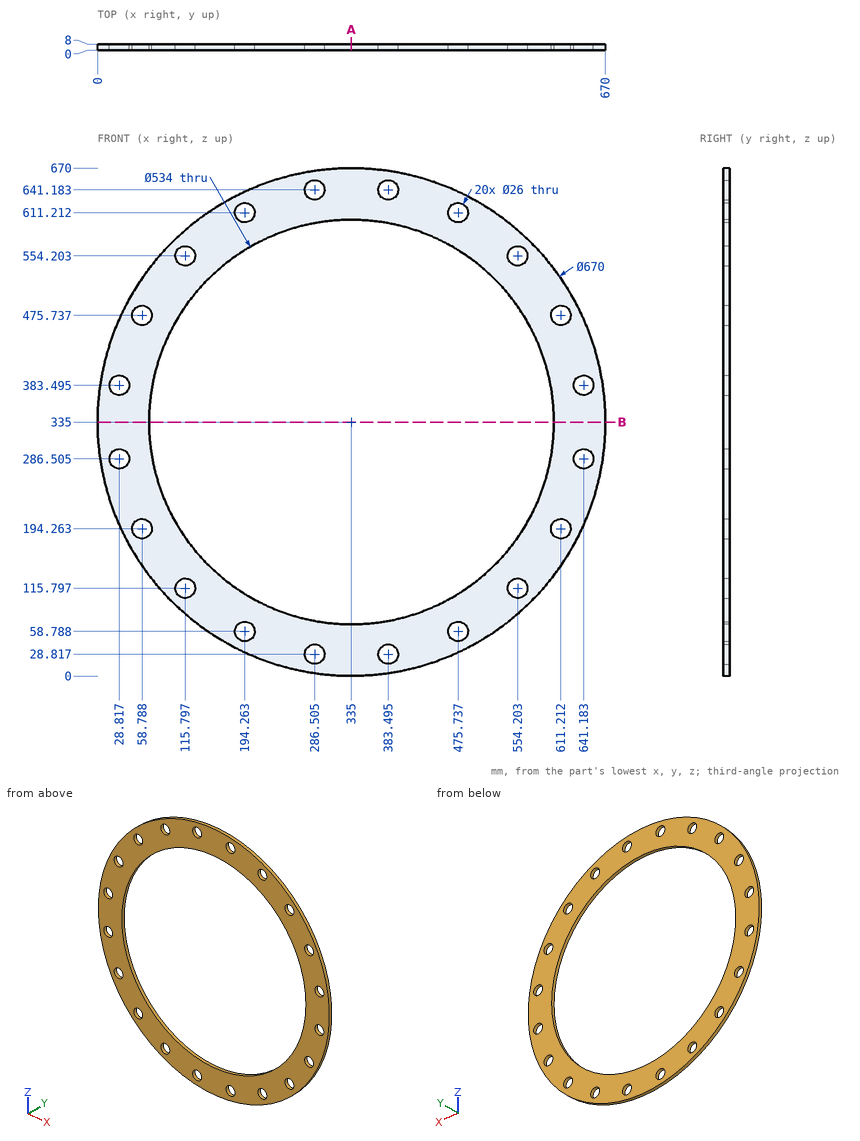
The figure shows three views and two pictorial views of one solid part (mm, origin at its lowest corner). Answer the questions. Give positions to 0.01 mm unless a question says otherwise; leave off trailing zeros. Loops run counter-clockwise (first coordinate to the right, second up) from the corner with the lowest first, then second, coordinate; pieces in that order, holes last. Notation, with made-up numbers: (71, -33.5) -> (97, -33.5) arc R9 ccw to (97, -29.5) -> close; hole circle Ø3 at (34.25, 31.25). An arc over 180 degrees is marked (long way). Put each result on its own line as item: value. Start each with the question number.
Item 1: The part is cut by section A-A (x = 335). Give the vertices of the cut face in (y, z).
Item 2: Find the intervals of material crossed by L1, parallel to X at y = 5, z = 634 (1 decimal); L2, parallel to Z at x = 335, y = 5; L3, parallel to Z at x = 58, y = 5.25 (1 decimal), in increasing order. Write a range as [from, to].
Item 3: The part is cut by section B-B (z = 335). Give the vertices of the cut face in (x, y).
Item 4: Each of these flat-tipped pins is pushed along its axis until it touches: P1, Ø2, axis at y = 1.5, z = 105, coming from the +X side; P2, Ø3, axis at y = 5, z = 365, coming from the -X side (1 decimal); P3, Ø1, axis at x = 147, z = 597, coming from the -Y side; P4, Ø2, axis at x = 398, y = 6, coming from the +Z side. Where does it stop, or does it pass through?
Answers below:
1. outline: (0, 0) -> (8, 0) -> (8, 68) -> (0, 68) -> close; (0, 602) -> (8, 602) -> (8, 670) -> (0, 670) -> close
2. L1: [183.9, 275.7], [297.3, 372.7], [394.3, 486.1]
2. L2: [0, 68], [602, 670]
2. L3: [146.6, 181.3], [207.2, 462.8], [488.7, 523.4]
3. outline: (0, 0) -> (68, 0) -> (68, 8) -> (0, 8) -> close; (602, 0) -> (670, 0) -> (670, 8) -> (602, 8) -> close
4. P1: x = 579.51
4. P2: x = 1.2
4. P3: y = 0
4. P4: z = 664.21
